Design review of the part built by this model. Coordinates are the model's own, in mm. A direction names the side the tool comes from. Give positions to 0.01 mm unless a question says otherwise; leave off trailing zeros. Loops run counter-clockwise (first coordinate to the right, second up) from the corner with the lowest first, then second, coordinate; pieces in that order, holes last. Notation, with made-up numbers: (59, 61) -> (106, 61) arc R6 ccw to (106, 68) -> close; hole circle Ø6 at (-8, 34). An arc over 180 degrees is marked (long way). Answer as CSV lines item,"result".
from build123d import *

# Parameters (mm, degrees)
PAD_DEPTH       = 42
SKETCH001_R     = 1.8
POCKET_DEPTH    = 6
SKETCH002_R     = 1.8
POCKET001_DEPTH = 4


with BuildPart() as part:
    # Sketch → Pad (new body)
    with BuildSketch(Plane.XY):
        Polygon((-21, 31), (2, 31), (2, 0), (-2, 0), (-2, 25), (-21, 25), align=None)
    extrude(amount=PAD_DEPTH)

    # Sketch001 → Pocket (cut)
    with BuildSketch(Plane(origin=(0, 31, 0), x_dir=(-1, 0, 0), z_dir=(0, 1, 0))):
        with Locations((6, 29)):
            Circle(SKETCH001_R)
        with Locations((18, 29)):
            Circle(SKETCH001_R)
        with Locations((6, 13)):
            Circle(SKETCH001_R)
        with Locations((18, 13)):
            Circle(SKETCH001_R)
    extrude(amount=-POCKET_DEPTH, mode=Mode.SUBTRACT)

    # Sketch002 → Pocket001 (cut)
    with BuildSketch(Plane(origin=(-2, 0, 0), x_dir=(0, -1, 0), z_dir=(-1, 0, 0))):
        with Locations((-4.241278, 34.5)):
            Circle(SKETCH002_R)
        with Locations((-4.241278, 7.5)):
            Circle(SKETCH002_R)
    extrude(amount=-POCKET001_DEPTH, mode=Mode.SUBTRACT)


solid = part.part
Q1. We need section C-C, the plane z = 7.5. State the section outline as (x, y) points.
Filled sheet:
outline,"(-21, 25) -> (-2, 25) -> (-2, 6.04) -> (2, 6.04) -> (2, 31) -> (-21, 31) -> close; (-2, 0) -> (2, 0) -> (2, 2.44) -> (-2, 2.44) -> close"
Q2. We need section D-D, the plane y = 7.5. State the section outline as (x, z) points.
Filled sheet:
outline,"(-2, 0) -> (2, 0) -> (2, 42) -> (-2, 42) -> close"
Q3. The part is to be moulded in two halves that separate along Z. For faces 1 (the flat face through (-2, 12, 21)), 2 (the flat face through (-1.7, 22.6, 0)), 3 (the cylindrical face through (-7.717, 28.042, 13.541)), say which applies: pulls with the +Z half, pulls with the -Z half, needs draft (parallel to the pull), parting line crosses it, or undercut.
Filled sheet:
face 1,"needs draft"
face 2,"pulls with the -Z half"
face 3,"undercut"
Q4. For faces 4 (the flat face through (0, 0, 21)), 5 (the flat face through (-11, 25, 21)), list the 3-axis set-ups (+Z, -Z, +X, -X, +Y, -Y) from which the entire face can be reached by the end or side of a thin tool; tool diameter is ignored.
Filled sheet:
face 4,"+Z, -Z, +X, -X, -Y"
face 5,"+Z, -Z, -X, -Y"
Q5. Clearance check with flat-ended pins moving along their axes: pin 1 Ø6 at (y, z) = (18.5, 25) entering from -X; pin 2 Ø6 at (x, z) = (-18, 29) entering from -Y; pin 3 Ø2 at (y, z) = (4.24, 34.5) entering from +X. State where each tip first meets the part, or that it passes through.
Filled sheet:
pin 1,"stops at x = -2"
pin 2,"stops at y = 25"
pin 3,"passes through"
Q6. We need section B-B, the plane z = 13. State the section outline as (x, y) points, and give its area (3 significant figures).
Filled sheet:
outline,"(-21, 25) -> (-19.8, 25) -> (-19.8, 31) -> (-21, 31) -> close; (-16.2, 25) -> (-7.8, 25) -> (-7.8, 31) -> (-16.2, 31) -> close; (-4.2, 25) -> (-2, 25) -> (-2, 0) -> (2, 0) -> (2, 31) -> (-4.2, 31) -> close"
area,"195 mm^2"
Q7. We need section A-A, the plane x = -18. State the section outline as (y, z) points, and give its area (3 significant figures).
Filled sheet:
outline,"(25, 0) -> (31, 0) -> (31, 11.2) -> (25, 11.2) -> close; (25, 14.8) -> (31, 14.8) -> (31, 27.2) -> (25, 27.2) -> close; (25, 30.8) -> (31, 30.8) -> (31, 42) -> (25, 42) -> close"
area,"209 mm^2"
Q8. To check wall thickness, follow probe 1 along Z at (x, y) = (-6, 26.7); probe 2 along Y at (x, z) = (-9.5, 29); probe 3 along X at (y, z) = (2, 19). State the ranges of each line that lie inside material, in increasing order. Write a range as from..to.
Filled sheet:
probe 1,"z = 0..11.2, 14.8..27.2, 30.8..42"
probe 2,"y = 25..31"
probe 3,"x = -2..2"
